Input: part model. Units: mm. Frame: model coordinates. A direction names the side the tool comes from. Coordinates: 2 decimals unless noted, no trailing zeros. Order: outer loops, then holes, each group sorted by start corner. A loop starts at its lowest first (then second) coordinate and runs counter-clockwise, first axis right, second up. Notation, with made-up numbers: M -18,89.25 L 30,89.25 A21 cw 30,97.25 Z; hole C -22.75,0 d11. An arc over 180 degrees is marked long. Answer in a Markdown table with one row per item.
from build123d import *

# Parameters (mm, degrees)
SKETCH_W        = 59.8
SKETCH_H        = 1.5
PAD_DEPTH       = 27.8
SKETCH002_W     = 52
SKETCH002_H     = 3
SKETCH002_W_2   = 30
SKETCH002_H_2   = 30
SKETCH002_W_3   = 4.6
SKETCH002_H_3   = 36
POCKET_DEPTH    = 5
SKETCH003_W     = 3.5
SKETCH003_H     = 6
PAD001_DEPTH    = 6
SKETCH004_R     = 1.75
POCKET001_DEPTH = 5


with BuildPart() as part:
    # Sketch → Pad (new body, symmetric)
    with BuildSketch(Plane.XZ):
        with Locations((0, 0.75)):
            Rectangle(SKETCH_W, SKETCH_H)
    extrude(amount=PAD_DEPTH, both=True)

    # Sketch002 → Pocket (cut)
    with BuildSketch(Plane(origin=(0, 0, 1.5), x_dir=(-1, 0, 0), z_dir=(0, 0, 1))):
        with Locations((0, 23.65)):
            Rectangle(SKETCH002_W, SKETCH002_H)
        with Locations((0, -23.65)):
            Rectangle(SKETCH002_W, SKETCH002_H)
        Rectangle(SKETCH002_W_2, SKETCH002_H_2)
        with Locations((24.6, 0)):
            Rectangle(SKETCH002_W_3, SKETCH002_H_3)
    extrude(amount=-POCKET_DEPTH, mode=Mode.SUBTRACT)

    # Sketch003 → Pad001 (new body)
    with BuildSketch(Plane(origin=(0, 0, 1.5), x_dir=(-1, 0, 0), z_dir=(0, 0, 1))):
        with Locations((-28.15, 26)):
            Rectangle(SKETCH003_W, SKETCH003_H)
        with Locations((-28.15, -26)):
            Rectangle(SKETCH003_W, SKETCH003_H)
    extrude(amount=PAD001_DEPTH)

    # Sketch004 → Pocket001 (cut)
    with BuildSketch(Plane(origin=(-26, 0, 0), x_dir=(0, 0, 1), z_dir=(1, 0, 0))):
        with Locations((-4.5, -25.5)):
            Circle(SKETCH004_R)
        with Locations((-4.5, 25.5)):
            Circle(SKETCH004_R)
    extrude(amount=-POCKET001_DEPTH, mode=Mode.SUBTRACT)


solid = part.part
1) Mould query, pull axis Y, two halves, no side actions, for faces 1 (the face through (-26.9, 0, 1)), 2 (the face through (0, 27.8, 1)), 3 (the face through (28, -26, 7.5)). Classes: +Y half, -Y half, draft (parallel to the pull), parting line (faces both ways), or undercut.
Resolved:
| item | result |
|---|---|
| face 1 | undercut |
| face 2 | +Y half |
| face 3 | draft |
2) Cut plane D-D, the plane x = -2. Output: boundary loops of the cut face in (y, z), and give its area (3 significant figures).
Resolved:
| item | result |
|---|---|
| outline | M -27.8,0 L -25.15,0 L -25.15,1.5 L -27.8,1.5 Z; M -22.15,0 L -15,0 L -15,1.5 L -22.15,1.5 Z; M 15,0 L 22.15,0 L 22.15,1.5 L 15,1.5 Z; M 25.15,0 L 27.8,0 L 27.8,1.5 L 25.15,1.5 Z |
| area | 29.4 mm2 |
3) Cut plane B-B, the plane y = 8.5. Output: boundary loops of the cut face in (x, z), and give its area (3 significant figures).
Resolved:
| item | result |
|---|---|
| outline | M -29.9,0 L -26.9,0 L -26.9,1.5 L -29.9,1.5 Z; M -22.3,0 L -15,0 L -15,1.5 L -22.3,1.5 Z; M 15,0 L 29.9,0 L 29.9,1.5 L 15,1.5 Z |
| area | 37.8 mm2 |
4) Cut plane A-A, the plane x = 17. Output: boundary loops of the cut face in (y, z), and give its area (3 significant figures).
Resolved:
| item | result |
|---|---|
| outline | M -27.8,0 L -25.15,0 L -25.15,1.5 L -27.8,1.5 Z; M -22.15,0 L 22.15,0 L 22.15,1.5 L -22.15,1.5 Z; M 25.15,0 L 27.8,0 L 27.8,1.5 L 25.15,1.5 Z |
| area | 74.4 mm2 |
5) Cut plane C-C, the plane z = 3.75. Output: boundary loops of the cut face in (x, y), and give its area (3 significant figures).
Resolved:
| item | result |
|---|---|
| outline | M 26.4,-29 L 29.9,-29 L 29.9,-23 L 26.4,-23 Z; M 26.4,23 L 29.9,23 L 29.9,29 L 26.4,29 Z |
| area | 42.0 mm2 |
6) Contact query for flat-ended pins moving along their axis: pin 1 (1.2 mm diameter, centred on x = 2, z = 0.5, fed in from -Y); pin 2 (1.6 mm diameter, centred on x = -8.5, z = 0.5, fed in from +Y); pin 3 (2 mm diameter, centred on y = -13, z = 3, fed in from -X). Output: stop coordinate, or through.
Resolved:
| item | result |
|---|---|
| pin 1 | stops at y = -27.8 |
| pin 2 | stops at y = 27.8 |
| pin 3 | passes through |
7) Reachability of faces 4 (the face through (29.9, 0, 1)), 5 (the face through (28, -23, 4)), 6 (the face through (0, 25.15, 1)) from +Z, -Z, +X, -X, +Y, -Y: full face, straight path, thin tool, end or side. Return the list, or none.
Resolved:
| item | result |
|---|---|
| face 4 | +Z, -Z, +X, +Y, -Y |
| face 5 | +Z, +X, -X |
| face 6 | +Z, -Z |
8) Material intervals for probe 1 along Y at (x, z) = (19, 1); probe 2 along X at (y, z) = (11, 0.75); probe 3 along Y at (x, z) = (-3, 0.5), sorted ascending.
Resolved:
| item | result |
|---|---|
| probe 1 | y = -27.8 to -25.15, -22.15 to 22.15, 25.15 to 27.8 |
| probe 2 | x = -29.9 to -26.9, -22.3 to -15, 15 to 29.9 |
| probe 3 | y = -27.8 to -25.15, -22.15 to -15, 15 to 22.15, 25.15 to 27.8 |
